The listing builds one solid part. Answer for the finished solid, in the listing's coordinates (mm). Face numbers are marked on the shaded views. A direction names the side the tool comes from. Coordinates: 2 decimals unless noted, no trailing zeros. Loops run counter-clockwise (first coordinate to the right, second up) from the corner with the lowest first, then second, coordinate; pieces in that order, holes last. Notation, with made-up numbers: M 16.25,73 L 60.25,73 A36 cw 60.25,107 Z; hole C 55,-0.75 d3. An arc over 180 degrees is marked long. Answer as CSV lines item,"result". Start each with the question number.
```python
from build123d import *

# Parameters (mm, degrees)
ESQUISSE1_W             = 30
ESQUISSE1_H             = 12
BOSS_EXTRU_1_DEPTH      = 2
ESQUISSE2_R             = 3.25
BOSS_EXTRU_2_DEPTH      = 0.5
ESQUISSE3_R             = 2.4
BOSS_EXTRU_3_DEPTH      = 4.2
ESQUISSE6_W             = 6.7
ESQUISSE6_H             = 31
BOSS_EXTRU_4_DEPTH      = 4.2
ESQUISSE8_W             = 4.2
ESQUISSE8_H             = 19
BOSS_EXTRU_5_DEPTH      = 2
ESQUISSE9_R             = 2.5
ENL_V_MAT_EXTRU_1_DEPTH = 4.2
CONG_1_R                = 3


with BuildPart() as part:
    # Esquisse1 → Boss.-Extru.1 (new body)
    with BuildSketch(Plane.XY):
        with Locations((2.190701098, -1.023529412)):
            Rectangle(ESQUISSE1_W, ESQUISSE1_H)
    extrude(amount=BOSS_EXTRU_1_DEPTH)

    # Esquisse2 → Boss.-Extru.2 (add)
    with BuildSketch(Plane.XY.offset(2)):
        with Locations((8.190701098, -1.023529412)):
            Circle(ESQUISSE2_R)
        with Locations((-3.809298902, -1.023529412)):
            Circle(ESQUISSE2_R)
    extrude(amount=BOSS_EXTRU_2_DEPTH)

    # Esquisse3 → Boss.-Extru.3 (add)
    with BuildSketch(Plane.XY.offset(2.5)):
        with Locations((-3.809298902, -1.023529412)):
            Circle(ESQUISSE3_R)
        with Locations((8.190701098, -1.023529412)):
            Circle(ESQUISSE3_R)
    extrude(amount=BOSS_EXTRU_3_DEPTH)

    # Esquisse6 → Boss.-Extru.4 (add)
    with BuildSketch(Plane(origin=(17.190701098, 0, 0), x_dir=(0, 0, -1), z_dir=(1, 0, 0))):
        with Locations((-3.35, -10.523529412)):
            Rectangle(ESQUISSE6_W, ESQUISSE6_H)
    extrude(amount=BOSS_EXTRU_4_DEPTH)

    # Esquisse8 → Boss.-Extru.5 (add)
    with BuildSketch(Plane.XY.offset(6.7)):
        with Locations((19.290701098, -16.523529412)):
            Rectangle(ESQUISSE8_W, ESQUISSE8_H)
    extrude(amount=BOSS_EXTRU_5_DEPTH)

    # Esquisse9 → Enlèv. mat.-Extru.1 (cut)
    with BuildSketch(Plane.ZY.offset(-17.190701098)):
        with Locations(Location((4.35, -17.023529412, 0), (0, 0, 270))):
            Circle(ESQUISSE9_R)
    extrude(amount=-ENL_V_MAT_EXTRU_1_DEPTH, mode=Mode.SUBTRACT)

    # Congé1
    cong_1_edges = [part.edges().sort_by_distance(p)[0] for p in [
        (19.290701098, -26.023529412, 0),
        (21.390701098, 4.976470588, 3.35),
        (19.290701098, -26.023529412, 8.7),
        (-12.809298902, 4.976470588, 1),
        (-12.809298902, -7.023529412, 1),
    ]]
    fillet(cong_1_edges, radius=CONG_1_R)


solid = part.part
```
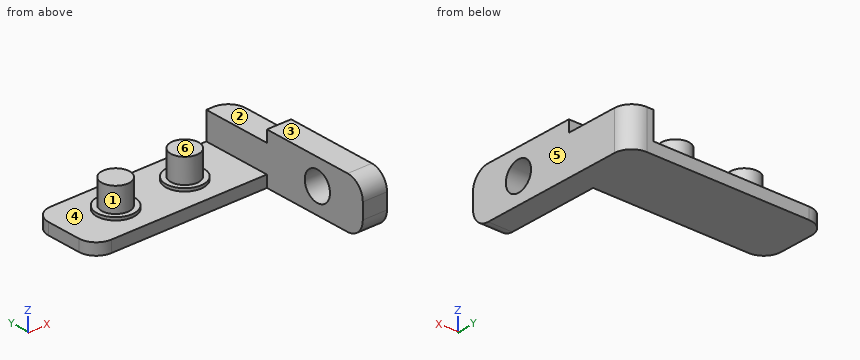
Item 1: Each of these flat-tipped pins is pushed along its axis until it touches: P1, Ø6, axis at x = 4, y = -1.5, coming from the +Z side; P2, Ø2.5, axis at y = -13.5, z = 3.5, coming from the -X side; P3, Ø2, axis at x = 19.5, z = 8, coming from the +Y side. Where does it stop, or does it pass through?
Item 2: Section A-A on x = 18 is taken. Determine the outline of the cut face in (y, z), then the cut area to 3 significant figures.
Item 3: Section B-B on z = 5.25 is taken. Determine the outline of the cut face in (x, y).
Item 4: For the marked faces 1, 2 and 3, determine the directions among +Z, -Z, +X, -X, +Y, -Y from which every point of the face is accessible in a straight line to the end or side of a thin tool.
Item 5: For a pull along X with two mould halves and no side action, classify the marked faces 4, 5 and 6 as pulls with the +X half, pulls with the -X half, needs draft (parallel to the pull), parting line crosses it, or undercut.
Item 6: Consider line 1 (X direction, y = -1, z = 5); line 2 (X direction, y = -2, z = 3); line 3 (X direction, y = -16, z = 0.75). Determine where each line is inside the solid, lowest interval first.
Item 7: Section D-D on z = 1.25 is taken. Determine the outline of the cut face in (x, y), then the cut area to 3 significant figures.
Item 8: Section C-C on x = -9 is taken. Determine the outline of the cut face in (y, z).
Results are:
1,P1,"z = 6.7"
1,P2,"x = 17.19"
1,P3,"y = -7.02"
2,outline,"M -26.02,3 A3 ccw -23.02,0 L 4.98,0 L 4.98,6.7 L -7.02,6.7 L -7.02,8.7 L -23.02,8.7 A3 ccw -26.02,5.7 Z; hole C -17.02,4.35 d5"
2,area,"222 mm²"
3,outline,"C -3.81,-1.02 d4.8; C 8.19,-1.02 d4.8; M 17.19,-26.02 L 21.39,-26.02 L 21.39,-19.36 L 17.19,-19.36 Z; M 17.19,-14.69 L 21.39,-14.69 L 21.39,1.98 A3 ccw 18.39,4.98 L 17.19,4.98 Z"
4,face 1,"+Z"
4,face 2,"+Z, +X, -X, +Y"
4,face 3,"+Z, +X, -X, +Y, -Y"
5,face 4,"undercut"
5,face 5,"pulls with the +X half"
5,face 6,"needs draft"
6,line 1,"-6.21 to -1.41, 5.79 to 10.59, 17.19 to 21.39"
6,line 2,"-6 to -1.62, 6 to 10.38, 17.19 to 21.39"
6,line 3,"17.19 to 21.39"
7,outline,"M -12.81,-4.02 A3 ccw -9.81,-7.02 L 17.19,-7.02 L 17.19,-25.46 L 21.39,-25.46 L 21.39,1.98 A3 ccw 18.39,4.98 L -9.81,4.98 A3 ccw -12.81,1.98 Z"
7,area,"482 mm²"
8,outline,"M -7.02,0 L 4.98,0 L 4.98,2 L -7.02,2 Z"
